from build123d import *

# Parameters (mm, degrees)
SKETCH1_W           = 58
SKETCH1_H           = 35
BOSS_EXTRUDE1_DEPTH = 1.5
BOSS_EXTRUDE2_DEPTH = 3
SKETCH4_R           = 4.5
SKETCH4_R_2         = 1.6
CUT_EXTRUDE1_DEPTH  = 55
CIRPATTERN1_COUNT   = 4
SKETCH5_R           = 3.05
CUT_EXTRUDE2_DEPTH  = 3
SKETCH6_R           = 2
CUT_EXTRUDE3_DEPTH  = 3
CIRPATTERN2_COUNT   = 4
FILLET1_SIZE        = 10
FILLET1_SIZE_2      = 15
SKETCH8_R           = 4
CUT_EXTRUDE4_DEPTH  = 3


with BuildPart() as part:
    # Sketch1 → Boss-Extrude1 (new, symmetric)
    with BuildSketch(Plane(origin=(0, 0, 0), x_dir=(1, 0, 0), z_dir=(0, 1, 0))):
        Rectangle(SKETCH1_W, SKETCH1_H)
    extrude(amount=BOSS_EXTRUDE1_DEPTH, both=True)

    # Sketch3 → Boss-Extrude2 (add)
    with BuildSketch(Plane.ZY.offset(29)):
        with BuildLine():
            Line((-17.5, 1.5), (-12.417185733, 45.436488243))
            ThreePointArc((-12.417185733, 45.436488243), (0, 56.5), (12.417185733, 45.436488243))
            Line((12.417185733, 45.436488243), (17.5, 1.5))
            Line((17.5, 1.5), (-17.5, 1.5))
        make_face()
    boss_extrude2 = extrude(amount=-BOSS_EXTRUDE2_DEPTH)

    # Sketch4 → Cut-Extrude1 (cut)
    with BuildSketch(Plane.ZY.offset(29)):
        with Locations((0, 44)):
            Circle(SKETCH4_R)
        with Locations((0, 51.2)):
            Circle(SKETCH4_R_2)
    cut_extrude1 = extrude(amount=-CUT_EXTRUDE1_DEPTH, mode=Mode.SUBTRACT)

    # CirPattern1: Cut-Extrude1 ×4 about axis
    cirpattern1_axis = Axis((0, 44, 0), (1, 0, 0))
    for i in range(1, CIRPATTERN1_COUNT):
        add(cut_extrude1.rotate(cirpattern1_axis, i * 360 / CIRPATTERN1_COUNT), mode=Mode.SUBTRACT)

    # Mirror1: Boss-Extrude2 across plane
    add(boss_extrude2.mirror(Plane(origin=(0, 0, 0), x_dir=(0, 0, 1), z_dir=(1, 0, 0))))

    # Sketch5 → Cut-Extrude2 (cut)
    with BuildSketch(Plane(origin=(0, 1.5, 0), x_dir=(1, 0, 0), z_dir=(0, 1, 0))):
        with Locations(Location((0, 0, 0), (0, 0, 270))):
            Circle(SKETCH5_R)
    extrude(amount=-CUT_EXTRUDE2_DEPTH, mode=Mode.SUBTRACT)

    # Sketch6 → Cut-Extrude3 (cut)
    with BuildSketch(Plane(origin=(0, 1.5, 0), x_dir=(1, 0, 0), z_dir=(0, 1, 0))):
        with Locations(Location((0, 12.5, 0), (0, 0, 270))):
            Circle(SKETCH6_R)
    cut_extrude3 = extrude(amount=-CUT_EXTRUDE3_DEPTH, mode=Mode.SUBTRACT)

    # CirPattern2: Cut-Extrude3 ×4 about axis
    cirpattern2_axis = Axis((0, 0, 0), (0, 1, 0))
    for i in range(1, CIRPATTERN2_COUNT):
        add(cut_extrude3.rotate(cirpattern2_axis, i * 360 / CIRPATTERN2_COUNT), mode=Mode.SUBTRACT)

    # Fillet1
    # an asymmetric fillet: 15, 10 mm, written as the material it adds along each edge
    with BuildSketch(Plane(origin=(-26, 1.5, 17.5), x_dir=(1, 0, 0), z_dir=(0, 0, -1))) as fillet1_piece_1_section:
        with BuildLine():
            Bezier((FILLET1_SIZE, 0), (0, 0), (0, -FILLET1_SIZE_2), weights=[1, 0.707106781, 1])
            Line((0, -FILLET1_SIZE_2), (0, 0))
            Line((0, 0), (FILLET1_SIZE, 0))
        make_face()
    fillet1_piece_1 = extrude(amount=35, mode=Mode.PRIVATE)
    fillet1_piece_1 = split(fillet1_piece_1, bisect_by=Plane(origin=(-23.803649904, 6.92315613, -16.872619514), z_dir=(0, -0.11491905943987848, 0.9933748586397049)), keep=Keep.TOP, mode=Mode.PRIVATE)
    fillet1_piece_1 = split(fillet1_piece_1, bisect_by=Plane(origin=(-23.803649904, 6.923154429, 16.872619711), z_dir=(0, -0.1149190594398785, -0.9933748586397049)), keep=Keep.TOP, mode=Mode.PRIVATE)
    add(fillet1_piece_1)
    with BuildSketch(Plane(origin=(26, 1.5, 17.5), x_dir=(-1, 0, 0), z_dir=(0, 0, -1))) as fillet1_piece_2_section:
        with BuildLine():
            Bezier((FILLET1_SIZE, 0), (0, 0), (0, FILLET1_SIZE_2), weights=[1, 0.707106781, 1])
            Line((0, FILLET1_SIZE_2), (0, 0))
            Line((0, 0), (FILLET1_SIZE, 0))
        make_face()
    fillet1_piece_2 = extrude(amount=35, mode=Mode.PRIVATE)
    fillet1_piece_2 = split(fillet1_piece_2, bisect_by=Plane(origin=(23.803649904, 6.92315613, -16.872619514), z_dir=(0, -0.11491905943987848, 0.9933748586397049)), keep=Keep.TOP, mode=Mode.PRIVATE)
    fillet1_piece_2 = split(fillet1_piece_2, bisect_by=Plane(origin=(23.803649904, 6.923154429, 16.872619711), z_dir=(0, -0.1149190594398785, -0.9933748586397049)), keep=Keep.TOP, mode=Mode.PRIVATE)
    add(fillet1_piece_2)

    # Sketch8 → Cut-Extrude4 (cut)
    with BuildSketch(Plane(origin=(29, 0, 0), x_dir=(0, 0, -1), z_dir=(1, 0, 0))):
        with Locations((0, 44)):
            Circle(SKETCH8_R)
    extrude(amount=-CUT_EXTRUDE4_DEPTH, mode=Mode.SUBTRACT)


solid = part.part
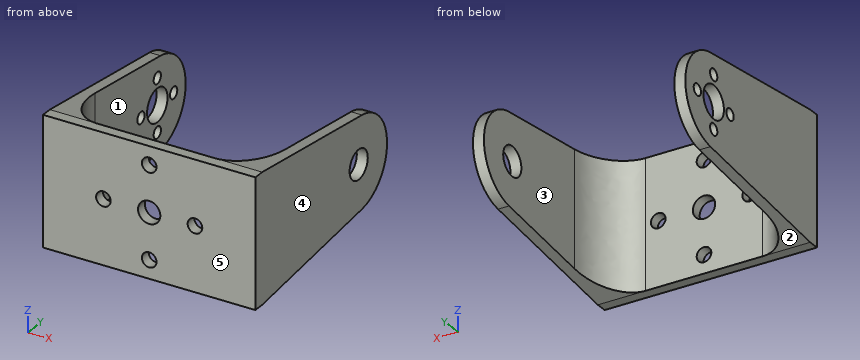
Read the model definition and answer for the solid it produces. Units are mm, in the model's axes. Face numbers are marked on the shaded views. A direction names the side the tool comes from. Coordinates: 2 decimals unless noted, no trailing zeros. Order: outer loops, then holes, each group sorted by start corner. A loop starts at its lowest first (then second) coordinate and runs counter-clockwise, first axis right, second up. Notation, with made-up numbers: (-12.75, 50.25) - (10.25, 50.25) arc R17 cw to (10.25, 65.25) - close; hole circle Ø1 at (26, 74). An arc over 180 degrees is marked (long way). Use one line per item in the form item = value.
(1) For a pull along X with two mould halves and no side action, classify the marked faces 3, 4 and 5 as pulls with the +X half, pulls with the -X half, needs draft (parallel to the pull), parting line crosses it, or undercut.
Computed values:
face_3 = undercut
face_4 = pulls with the +X half
face_5 = needs draft
(2) Section B-B, the plane y = 23 is taken. Give the vertices of the cut face in (x, z).
Computed values:
outline = (-29, -15.01) - (-26, -15.01) - (-26, 15.01) - (-29, 15.01) - close; (26, -15.01) - (29, -15.01) - (29, 15.01) - (26, 15.01) - close
(3) Given pin 1 Ø3.5 at (x, z) = (0, -12.5) entering from +Y; pin 2 Ø3 at (x, z) = (-6, -13) entering from +Y; pin 3 Ø2.5 at (y, z) = (36.8, 0) entering from -X, each flat-ended and moving along its own axis, determine where each tip first touches the part or whether it passes through.
Computed values:
pin_1 = through
pin_2 = 1.5
pin_3 = 26
(4) Section A-A, the plane x = 0 is taken. Give the vertices of the cut face in (y, z).
Computed values:
outline = (-1.5, -17.5) - (1.5, -17.5) - (1.5, -14.5) - (-1.5, -14.5) - close; (-1.5, -10.5) - (1.5, -10.5) - (1.5, -3.05) - (-1.5, -3.05) - close; (-1.5, 3.05) - (1.5, 3.05) - (1.5, 10.5) - (-1.5, 10.5) - close; (-1.5, 14.5) - (1.5, 14.5) - (1.5, 17.5) - (-1.5, 17.5) - close
(5) Straight lines are drawn through the part: L1, parallel to Y at x = -27.1, z = 0; L2, parallel to X at y = 53.5, z = 8; L3, parallel to Y at x = 27, z = 0. For each, find the intervals that lie inside material, in ascending order.
Computed values:
L1 = -1.5 to 35.2, 38.4 to 39.5, 48.5 to 49.6, 52.8 to 56.5
L2 = -29 to -26, 26 to 29
L3 = -1.5 to 40, 48 to 56.5
(6) Which of the six approach directions +Z, -Z, +X, -X, +Y, -Y give full straight-line access (tool end or side, diameter ignored) to the marked faces 1 and 2?
Computed values:
face_1 = +Z, -Z, +Y
face_2 = -Z, +X, -X, +Y
(7) Section D-D, the plane z = 0 is taken. Give the number of separate pieces and of enclosed holes in the cut face, then the cut area to 3 significant figures.
Computed values:
separate_pieces = 8
enclosed_holes = 0
area = 456 mm²
(8) Section C-C, the plane x = -12.5 is taken. Give the vertices of the cut face in (y, z).
Computed values:
outline = (-1.5, -17.5) - (1.5, -17.5) - (1.5, -2) - (-1.5, -2) - close; (-1.5, 2) - (1.5, 2) - (1.5, 17.5) - (-1.5, 17.5) - close
